Autodesk Inventor part; units mm, degrees
ref_plane "YZ Plane" through (0, 0, 0) normal (1, 0, 0) x (0, 1, 0)
ref_plane "XZ Plane" through (0, 0, 0) normal (0, 1, 0) x (-1, 0, 0)
ref_plane "XY Plane" through (0, 0, 0) normal (0, 0, 1) x (1, 0, 0)
sketch "Sketch1" plane through (0, 0, 0) normal (0, 1, 0) x (-1, 0, 0)
  line L0 (0, 0) -> (-50.8, 0)
  line L1 (-50.8, 0) -> (-50.8, -50.8)
  line L2 (-50.8, -50.8) -> (0, -50.8)
  line L3 (0, -50.8) -> (0, 0)
  line L4 (-50.8, 0) -> (-101.6, 0)
  line L5 (-101.6, 0) -> (-101.6, -25.4)
  line L6 (-101.6, -25.4) -> (-50.8, -25.4)
  line L7 (-50.8, -25.4) -> (-50.8, 0)
  line L8 (-50.8, 0) -> (-101.6, 0)
  line L9 (-101.6, 0) -> (-101.6, 2.2098)
  line L10 (-101.6, 2.2098) -> (-50.8, 2.2098)
  line L11 (-50.8, 2.2098) -> (-50.8, 0)
  dimension "d0" = 50.8
  dimension "d1" = 50.8
  dimension "d2" = 50.8
  dimension "d3" = 2.2098
extrude "Extrusion1" add sketch "Sketch1" against normal blind 2.2098
extrude "Extrusion2" add sketch "Sketch1" along normal blind 50.8 contours L4 L9 L10 L11
fillet "Fillet1" radius 2.2098 1 edges at (76.2, -2.2098, 2.2098)
sketch "Sketch2" plane through (0, 0, 0) normal (0, 1, 0) x (1, 0, 0)
  line L0 (50.8, 0) -> (101.6, 0)
  line L1 (101.6, 0) -> (101.6, 25.4)
  line L2 (101.6, 25.4) -> (50.8, 25.4)
  line L3 (50.8, 25.4) -> (50.8, 50.8)
  line L4 (50.8, 50.8) -> (0, 50.8)
  line L5 (0, 50.8) -> (0, 0)
  line L6 (0, 0) -> (50.8, 0)
  line L7 (10.1727, 10.1727) -> (40.6273, 10.1727)
  line L8 (40.6273, 10.1727) -> (40.6273, 40.6273)
  line L9 (40.6273, 40.6273) -> (10.1727, 40.6273)
  line L10 (10.1727, 40.6273) -> (10.1727, 10.1727)
  dimension "d9" = 30.4546
  dimension "d10" = 30.4546
hole "Hole1" at (10.1727, 0, -40.6273) at (10.1727, 0, -10.1727) at (40.6273, 0, -40.6273) at (40.6273, 0, -10.1727) direction (0, -1, 0) diameter 3.302 end through all
sketch "Sketch3" plane through (0, 0, 0) normal (0, 1, 0) x (1, 0, 0)
  line L0 (50.8, 0) -> (101.6, 0)
  line L1 (101.6, 0) -> (101.6, 33.655)
  line L2 (101.6, 33.655) -> (50.8, 33.655)
  line L3 (50.8, 33.655) -> (50.8, 0)
  line L4 (50.8, 33.655) -> (101.6, 33.655)
  line L5 (101.6, 33.655) -> (101.6, 59.055)
  line L6 (101.6, 59.055) -> (50.8, 59.055)
  line L7 (50.8, 59.055) -> (50.8, 33.655)
  point P0 (0, 0)
  dimension "d18" = 33.655
  dimension "d19" = 25.4
extrude "Extrusion3" cut sketch "Sketch3" against normal blind 25.4 contours L3 L2 L1 L0
extrude "Extrusion4" add sketch "Sketch3" against normal blind 2.2098 contours L7 L6 L5 L2
sketch "Sketch4" plane through (0, 50.8, 0) normal (0, 1, 0) x (1, 0, 0)
  point P0 (0, 0)
sketch "Sketch5" plane through (0, 50.8, 0) normal (0, 1, 0) x (1, 0, 0)
  line L0 (50.8, 0) -> (101.6, 0)
  line L1 (101.6, 0) -> (101.6, -2.2098)
  line L2 (101.6, -2.2098) -> (50.8, -2.2098)
  line L3 (50.8, -2.2098) -> (50.8, 0)
  point P0 (0, 0)
extrude "Extrusion5" cut sketch "Sketch5" against normal through all
sketch "Sketch7" plane through (0, -2.2098, 0) normal (0, -1, 0) x (1, 0, 0)
  line L0 (50.8, -33.655) -> (101.6, -33.655)
  line L1 (101.6, -33.655) -> (101.6, -31.4452)
  line L2 (101.6, -31.4452) -> (50.8, -31.4452)
  line L3 (50.8, -31.4452) -> (50.8, -33.655)
  point P0 (0, 0)
  dimension "d27" = 50.8
  dimension "d28" = 2.2098
extrude "Extrusion6" add sketch "Sketch7" against normal blind 53.0098
fillet "Fillet2" radius 2.2098 1 edges at (76.2, -2.2098, -31.4452)
sketch "Sketch8" plane through (0, 0, 0) normal (0, 1, 0) x (1, 0, 0)
  line L0 (50.8, 0) -> (50.8, 31.4452)
  line L1 (50.8, 31.4452) -> (50.8, 33.655)
  line L2 (50.8, 33.655) -> (101.6, 33.655)
  line L3 (101.6, 33.655) -> (101.6, 59.055)
  line L4 (101.6, 59.055) -> (50.8, 59.055)
  line L5 (50.8, 59.055) -> (50.8, 50.8)
  line L6 (50.8, 50.8) -> (0, 50.8)
  line L7 (0, 50.8) -> (0, 0)
  line L8 (0, 0) -> (50.8, 0)
  circle A0 centre (40.6273, 10.1727) radius 1.651
  circle A1 centre (10.1727, 10.1727) radius 1.651
  circle A2 centre (10.1727, 40.6273) radius 1.651
  circle A3 centre (40.6273, 40.6273) radius 1.651
  line L9 (50.8, 59.055) -> (101.6, 59.055)
  line L10 (101.6, 59.055) -> (101.6, 76.6318)
  line L11 (101.6, 76.6318) -> (50.8, 76.6318)
  line L12 (50.8, 76.6318) -> (50.8, 59.055)
  line L13 (50.8, 50.8) -> (0, 50.8)
  line L14 (0, 50.8) -> (0, 76.6318)
  line L15 (0, 76.6318) -> (50.8, 76.6318)
  line L16 (50.8, 76.6318) -> (50.8, 50.8)
  dimension "d32" = 17.5768
extrude "Extrusion7" add sketch "Sketch8" against normal blind 2.2098 contours L14 L15 L12 L5 L6 | L4 L12 L11 L10
sketch "Sketch9" plane through (0, 0, 0) normal (0, 1, 0) x (1, 0, 0)
  line L0 (101.6, 76.6318) -> (50.8, 76.6318)
  line L1 (50.8, 76.6318) -> (50.8, 51.2318)
  line L2 (50.8, 51.2318) -> (101.6, 51.2318)
  line L3 (101.6, 51.2318) -> (101.6, 76.6318)
  line L4 (50.8, 51.2318) -> (112.668, 51.2318)
  line L5 (112.668, 51.2318) -> (112.668, 0)
  line L6 (112.668, 0) -> (50.8, 0)
  line L7 (50.8, 0) -> (50.8, 51.2318)
  point P0 (0, 0)
  dimension "d35" = 25.4
extrude "Extrusion8" cut sketch "Sketch9" against normal blind 2.2098 contours L4 L5 L6 L7 L2
sketch "Sketch10" plane through (0, 50.8, 0) normal (0, 1, 0) x (1, 0, 0)
  line L0 (50.8, 33.655) -> (116.0287, 33.655)
  line L1 (116.0287, 33.655) -> (116.0287, 19.3076)
  line L2 (116.0287, 19.3076) -> (50.8, 19.3076)
  line L3 (50.8, 19.3076) -> (50.8, 33.655)
  point P0 (0, 0)
extrude "Extrusion9" cut sketch "Sketch10" against normal through all
sketch "Sketch11" plane through (0, 0, 0) normal (0, 1, 0) x (1, 0, 0)
  line L0 (50.8, 51.2318) -> (101.6, 51.2318)
  line L1 (101.6, 51.2318) -> (101.6, 76.6318)
  line L2 (101.6, 76.6318) -> (0, 76.6318)
  line L3 (0, 76.6318) -> (0, 0)
  line L4 (0, 0) -> (50.8, 0)
  line L5 (50.8, 0) -> (50.8, 51.2318)
  circle A0 centre (40.6273, 10.1727) radius 1.651
  circle A1 centre (10.1727, 10.1727) radius 1.651
  circle A2 centre (10.1727, 40.6273) radius 1.651
  circle A3 centre (40.6273, 40.6273) radius 1.651
  line L6 (50.8, 51.2318) -> (101.6, 51.2318)
  line L7 (101.6, 51.2318) -> (101.6, 49.022)
  line L8 (101.6, 49.022) -> (50.8, 49.022)
  line L9 (50.8, 49.022) -> (50.8, 51.2318)
  dimension "d40" = 2.2098
extrude "Extrusion10" add sketch "Sketch11" along normal blind 50.8 contours L0 L7 L8 L5
sketch "Sketch12" plane through (0, 0, 0) normal (0, -1, 0) x (1, 0, 0)
  line L0 (50.8, -51.2318) -> (50.8, -49.022)
  line L1 (101.6, -48.9148) -> (50.8, -48.9148)
  line L2 (50.8, -48.9148) -> (50.8, -51.1246)
  line L3 (50.8, -51.1246) -> (101.6, -51.1246)
  line L4 (101.6, -51.1246) -> (101.6, -48.9148)
  point P0 (0, 0)
  dimension "d43" = 2.2098
extrude "Extrusion11" add sketch "Sketch12" along normal blind 2.2098
fillet "Fillet3" radius 2.2098 1 edges at (76.2, -2.2098, -48.9148)
sketch "Sketch14" plane through (0, -2.2098, 0) normal (0, -1, 0) x (1, 0, 0)
  line L0 (101.6, -76.6318) -> (0, -76.6318)
  line L1 (0, -76.6318) -> (0, -78.8416)
  line L2 (0, -78.8416) -> (101.6, -78.8416)
  line L3 (101.6, -78.8416) -> (101.6, -76.6318)
  point P0 (0, 0)
  dimension "d47" = 2.2098
extrude "Extrusion12" add sketch "Sketch14" against normal blind 53.0098
sketch "Sketch15" plane through (101.6, -2.2098, -78.8416) normal (0, 0, -1) x (-1, 0, 0)
  line L0 (101.6, 53.0098) -> (0, 53.0098)
  line L1 (101.6, 2.2098) -> (50.8, 53.0098)
  line L2 (101.6, 2.2098) -> (101.6, 53.0098)
  line L3 (101.6, 2.2098) -> (101.6, 53.0098)
  line L4 (101.6, 53.0098) -> (50.8, 53.0098)
  dimension "d50" = 50.8
extrude "Extrusion13" cut sketch "Sketch15" against normal blind 2.2098
fillet "Fillet4" radius 2.2098 1 edges at (50.8, -2.2098, -78.8416)
sketch "Sketch16" plane through (0, 0, 0) normal (0, 1, 0) x (1, 0, 0)
  line L0 (0, 0) -> (50.8, 0)
  line L1 (50.8, 0) -> (50.8, 50.8)
  line L2 (50.8, 50.8) -> (0, 50.8)
  line L3 (0, 50.8) -> (0, 0)
  circle A0 centre (25.4, 25.4) radius 5.0038
  dimension "d54" = 50.8
  dimension "d55" = 10.0076
extrude "Extrusion14" cut sketch "Sketch16" against normal blind 3.175 contours A0
properties part number "Arm holder Bracket"
Here's how the part is built. I have some questions about the finished solid (model axes, mm). A direction names the side the tool comes from. Round coordinates to 2 decimals unless told otherwise and drop trailing zeros. Loops run counter-clockwise (first coordinate to the right, second up) from the corner with the lowest first, then second, coordinate; pieces in that order, holes last. Notation, with made-up numbers: (84, 79.25) - (116, 79.25) arc R29 cw to (116, 116.25) - close; hole circle Ø2 at (-26.5, -27). An arc over 180 degrees is marked (long way). One line per question, with ' | ' between items. Start each with the question number.
Q1. I want a section at A-A (y = 17.5). Write out the boundary of the cut face in (x, z), then the cut area to 3 significant figures.
Q2. Will these pins go through, and if not, where does the flat tip stop? pin 1 (4.5 mm diameter, centred on x = 10.17, z = -40.63, fed in from -Y); pin 2 (2 mm diameter, centred on x = 40, y = 36.5, fed in from +Z); pin 3 (4 mm diameter, centred on x = 10.17, z = -10.17, fed in from +Y); pin 4 (0.7 mm diameter, centred on y = -0.5, z = -16, fed in from +X).
Q3. I want a section at C-C (z = -25.4). Write out the boundary of the cut face in (x, y).
Q4. Please list where these lines run through material, in increasing order: line 1 (Z direction, x = 55, y = 46.5); line 2 (Y direction, x = 37, z = -16.5); line 3 (Y direction, x = 55, z = -51). Write a range as [from, to].
Q5. I want a section at B-B (x = 25.4). Write out the boundary of the cut face in (y, z).
Q6. I want a section at D-D (z = -40.5). Write out the boundary of the cut face in (x, y), then the cut area to 3 significant figures.
Q7. For faces 1 (the flat face through (77, 25, -49.022)), 2 (the cylindrical face through (75.8, -1.6, -49.6)), 3 (the flat face through (50.8, 25, -50)), 4 (the flat face through (76, 25, -51.232)), 5 (the flat face through (101.6, 25, -50)), which set-ups out of +Z, -Z, +X, -X, +Y, -Y let a thin tool reach every point of the face, with its end or its side?
Response values:
1) outline: (17.5, -78.84) - (101.6, -78.84) - (101.6, -76.63) - (17.5, -76.63) - close; (50.8, -51.23) - (101.6, -51.23) - (101.6, -49.02) - (50.8, -49.02) - close | area: 298 mm²
2) pin 1: stops at y = -2.21 | pin 2: stops at z = -76.63 | pin 3: stops at y = 0 | pin 4: stops at x = 50.8
3) outline: (0, -2.21) - (20.4, -2.21) - (20.4, 0) - (0, 0) - close; (30.4, -2.21) - (50.8, -2.21) - (50.8, 0) - (30.4, 0) - close
4) line 1: z = [-78.84, -76.63], [-51.23, -49.02] | line 2: y = [-2.21, 0] | line 3: y = [-2.21, 50.8]
5) outline: (-2.21, -76.63) arc R2.21 ccw to (0, -78.84) - (25.4, -78.84) - (25.4, -76.63) - (0, -76.63) - (0, -30.4) - (-2.21, -30.4) - close; (-2.21, -20.4) - (0, -20.4) - (0, 0) - (-2.21, 0) - close
6) outline: (0, -2.21) - (8.53, -2.21) - (8.53, 0) - (0, 0) - close; (11.82, -2.21) - (38.98, -2.21) - (38.98, 0) - (11.82, 0) - close; (42.27, -2.21) - (50.8, -2.21) - (50.8, 0) - (42.27, 0) - close | area: 97.7 mm²
7) face 1: +Z, +X, -X, +Y | face 2: +Z, +X, -Y | face 3: +Z, -X, +Y | face 4: +X, -X, +Y | face 5: +Z, -Z, +X, +Y, -Y
